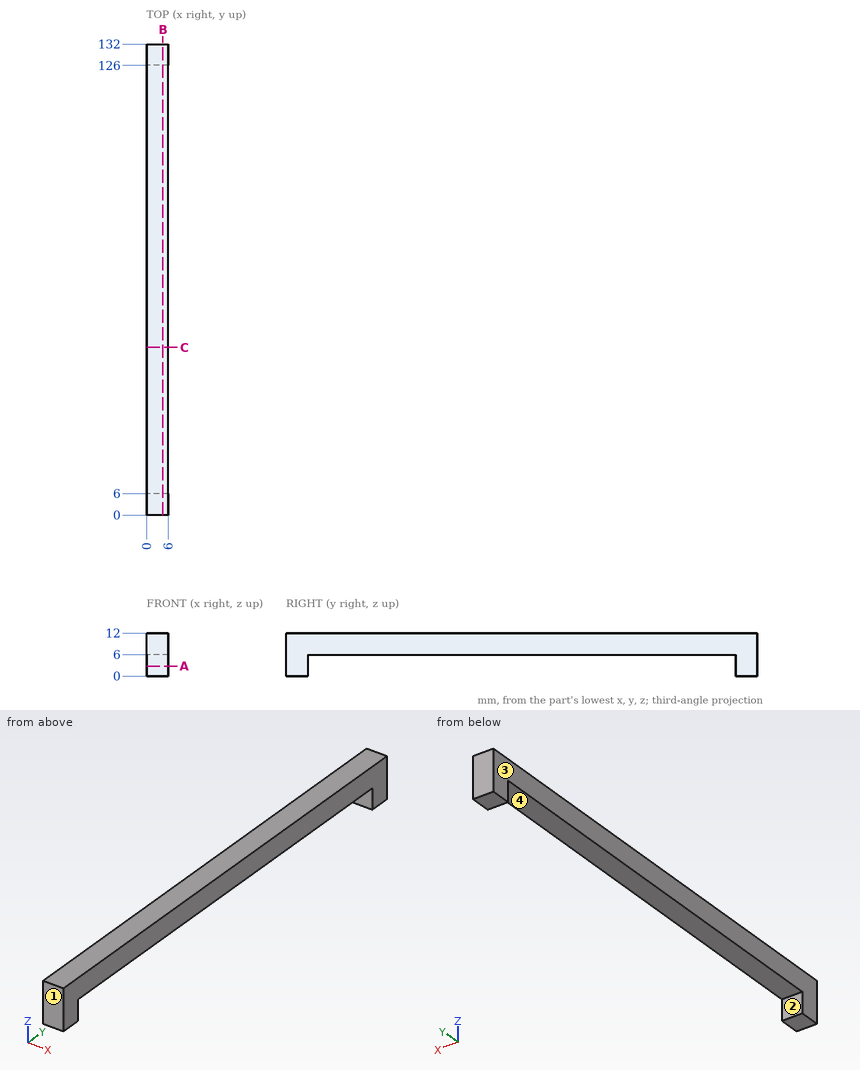
Print and shaded views of the part. All mm, measured from the part's lowest x, y and z. Coordinates: 2 decimals unless noted, no trailing zeros. Write each loop counter-clockwise with the first axis right and the second up, starting at its lowest first coordinate (ties: lowest second). Pieces come first, ordered by that corner, then holes. Notation, with made-up numbers: (73, 58.5) -> (102, 58.5) arc R23 cw to (102, 95.5) -> close; hole circle Ø11 at (79, 12.5). An arc over 180 degrees is marked (long way). Use CSV: the item, a comma, the result in double quotes. Start each with the question number.
Q1. Drill centre lines: probe 1 along Y at (x, z) = (4.15, 4.5); probe 2 along Z at (x, y) = (1.45, 87.5). Where is each one in solid material? Low to high.
Q2. Cut at C-C, the plane y = 47. List the corners of the cut face in (x, z).
Q3. Cut at A-A, the plane z = 2.75. List the corners of the cut face in (x, y), then the cut area to 3 significant figures.
Q4. Pull direction Y, two halves, no side cores. Call the marked faces 1, 2, 3 and 4: released by +Y, released by -Y, zero draft, split by the parting line, or undercut.
Q5. Cut at B-B, the plane x = 4.55. List the corners of the cut face in (y, z), then the cut area to 3 significant figures.
Checked values:
1,probe 1,"y = 0 to 6, 126 to 132"
1,probe 2,"z = 6 to 12"
2,outline,"(0, 6) -> (6, 6) -> (6, 12) -> (0, 12) -> close"
3,outline,"(0, 0) -> (6, 0) -> (6, 6) -> (0, 6) -> close; (0, 126) -> (6, 126) -> (6, 132) -> (0, 132) -> close"
3,area,"72.0 mm²"
4,face 1,"released by -Y"
4,face 2,"undercut"
4,face 3,"zero draft"
4,face 4,"undercut"
5,outline,"(0, 0) -> (6, 0) -> (6, 6) -> (126, 6) -> (126, 0) -> (132, 0) -> (132, 12) -> (0, 12) -> close"
5,area,"864 mm²"
